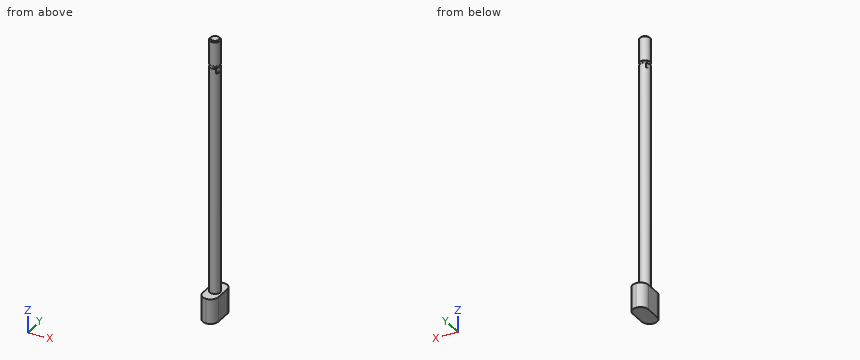
from build123d import *

# Parameters (mm, degrees)
SKETCH2_W           = 145.15
SKETCH2_H           = 3
CUT_EXTRUDE1_DEPTH  = 3.3
BOSS_EXTRUDE1_DEPTH = 14.3


with BuildPart() as part:
    # Sketch1 → Revolve1 (revolve)
    with BuildSketch(Plane(origin=(0, 0, 0), x_dir=(0, 0, -1), z_dir=(1, 0, 0))):
        with BuildLine():
            Line((-23, 0), (-23, 2.3865))
            Line((-23, 2.3865), (-22.3865, 3))
            Line((-22.3865, 3), (-8.5, 3))
            ThreePointArc((-8.5, 3), (-8.324264069, 2.575735931), (-7.9, 2.4))
            Line((-7.9, 2.4), (-7.6, 2.4))
            ThreePointArc((-7.6, 2.4), (-7.175735931, 2.575735931), (-7, 3))
            Line((-7, 3), (-6.5, 3))
            Line((-6.5, 3), (-6.5, 0))
            Line((-6.5, 0), (-23, 0))
        make_face()
    revolve(axis=Axis((0, 0, 6.5), (0, 0, 1)))

    # Sketch2 → Revolve2 (revolve)
    with BuildSketch(Plane(origin=(0, 0, 0), x_dir=(0, 0, -1), z_dir=(1, 0, 0))):
        with Locations((65.575, 1.5)):
            Rectangle(SKETCH2_W, SKETCH2_H)
    revolve(axis=Axis((0, 0, -138.15), (0, 0, 1)))

    # Sketch3 → Cut-Extrude1 (cut)
    with BuildSketch(Plane.XY.offset(4.3)):
        Polygon((-6.447248163, -4.742941189), (3.2120101, -7.33113164), (5.800200551, 2.328126623), (3.385385985, 2.975174236), (1.12071934, -5.476676744), (-3.708909791, -4.182581519), (-1.444243147, 4.269269461), (-3.859057712, 4.916317074), align=None)
    extrude(amount=CUT_EXTRUDE1_DEPTH, mode=Mode.SUBTRACT)

    # Sketch4 → Boss-Extrude1 (add)
    with BuildSketch(Plane.XY.offset(-138.15)):
        with BuildLine():
            Line((4.5, -4.5), (4.5, 4.5))
            ThreePointArc((4.5, 4.5), (3.181980515, 7.681980515), (0, 9))
            ThreePointArc((0, 9), (-3.181980515, 7.681980515), (-4.5, 4.5))
            Line((-4.5, 4.5), (-4.5, -4.5))
            ThreePointArc((-4.5, -4.5), (-3.181980515, -7.681980515), (0, -9))
            ThreePointArc((0, -9), (3.181980515, -7.681980515), (4.5, -4.5))
        make_face()
    extrude(amount=BOSS_EXTRUDE1_DEPTH)


solid = part.part
Verification items for the finished model (mm, model axes). Round coordinates to 2 decimals unless told otherwise and drop trailing zeros. Loops run counter-clockwise (first coordinate to the right, second up) from the corner with the lowest first, then second, coordinate; pieces in that order, holes last. Notation, with made-up numbers: (63.5, 40.5) - (97.5, 40.5) arc R20 ccw to (97.5, 47.5) - close; hole circle Ø5 at (48, -10.5). An arc over 180 degrees is marked (long way). Use a Markdown table: item, result. Add a question column.
1. Section check B-B, the plane y = -6.75. Record the boundary of the cut face in (x, z), plus the area to 3 significant figures.
2. Section check A-A, the plane z = -84.5. Record the boundary of the cut face in (x, y).
3. Thickness scan on probe 1 along Y at (x, z) = (-0.25, -50); probe 2 along Y at (x, z) = (2, -30); probe 3 along Z at (x, y) = (2.5, 6.75). Record the ranges inside material, lowest first. Write a range as [from, to].
4. Gauge pin test, flat ends, axial feed: pin 1 (1.5 mm diameter, centred on y = 0.5, z = -99, fed in from +X); pin 2 (0.5 mm diameter, centred on x = -2.5, y = 1, fed in from +Z); pin 3 (2 mm diameter, centred on x = 1.5, z = 4.5, fed in from +Y). Record the tip position at first contact, or that the pin passes through.
Checks:
| question | item | result |
|---|---|---|
| 1 | outline | (-3.9, -138.15) - (3.9, -138.15) - (3.9, -123.85) - (-3.9, -123.85) - close |
| 1 | area | 111 mm^2 |
| 2 | outline | circle Ø6 at (0, 0) |
| 3 | probe 1 | y = [-2.99, 2.99] |
| 3 | probe 2 | y = [-2.24, 2.24] |
| 3 | probe 3 | z = [-138.15, -123.85] |
| 4 | pin 1 | stops at x = 3 |
| 4 | pin 2 | stops at z = 22.94 |
| 4 | pin 3 | stops at y = 2.96 |
